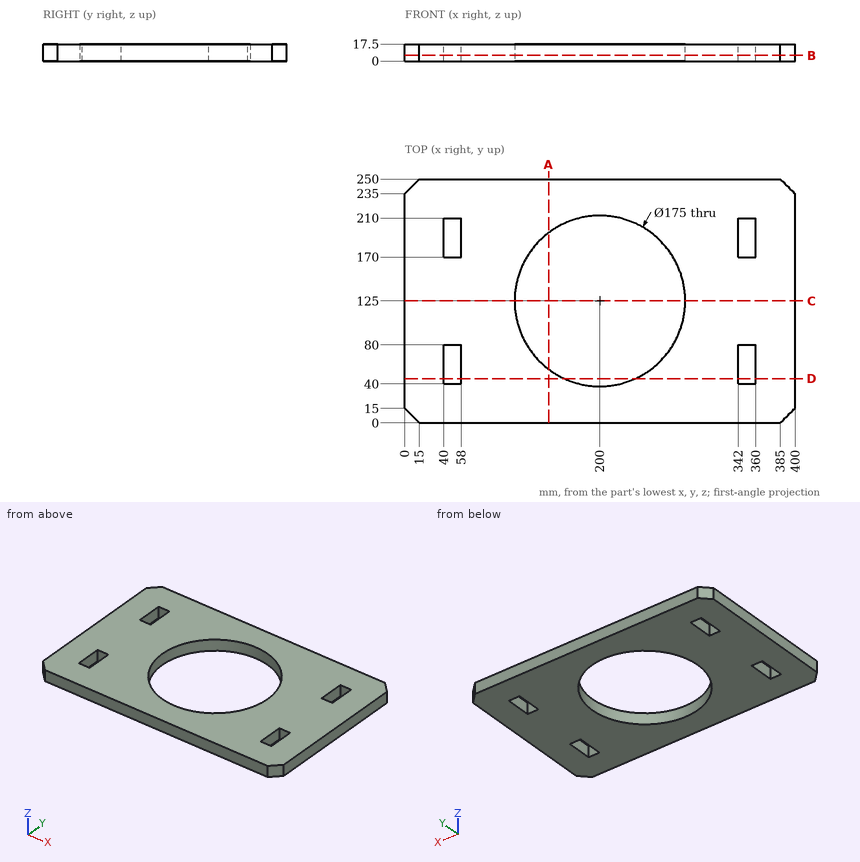
Answer from the drawing. Dimensions are ordinates in mm from the lowest x, y and z of the part. Round coordinates to 2 decimals unless told otherwise and drop trailing zeros. Write each loop counter-clockwise with the first axis right and the second up, starting at its lowest first coordinate (ties: lowest second). Pieces come first, ordered by that corner, then holes. Notation, with made-up numbers: M -18,-4 L 24,-4 A24 cw 24,26 Z; hole C -38.5,30 d6. An arc over 180 degrees is marked long. Write each question's results on one line, items separated by ' | '. Start each with the question number.
Item 1: A cutting plane is placed at B-B on z = 5.75. Write down the section's boundary in (x, y), and give its area (3 significant figures).
Item 2: A cutting plane is placed at C-C on y = 125. Write down the section's boundary in (x, z).
Item 3: A cutting plane is placed at A-A on x = 147.5. Write down the section's boundary in (y, z).
Item 4: A cutting plane is placed at D-D on y = 45.5. Write down the section's boundary in (x, z).
Item 5: Straight lines are drawn through the part: L1, parallel to Y at x = 50.5, z = 7; L2, parallel to X at y = 203, z = 11.5; L3, parallel to Y at x = 200, z = 9.75. For each, find the intervals that lie inside material, in ascending order. Write a range as [from, to].
Check sheet entries:
1) outline: M 0,15 L 15,0 L 385,0 L 400,15 L 400,235 L 385,250 L 15,250 L 0,235 Z; hole M 40,40 L 58,40 L 58,80 L 40,80 Z; hole M 40,170 L 58,170 L 58,210 L 40,210 Z; hole C 200,125 d175; hole M 342,40 L 360,40 L 360,80 L 342,80 Z; hole M 342,170 L 360,170 L 360,210 L 342,210 Z | area: 72,600 mm²
2) outline: M 0,0 L 112.5,0 L 112.5,17.5 L 0,17.5 Z; M 287.5,0 L 400,0 L 400,17.5 L 287.5,17.5 Z
3) outline: M 0,0 L 55,0 L 55,17.5 L 0,17.5 Z; M 195,0 L 250,0 L 250,17.5 L 195,17.5 Z
4) outline: M 0,0 L 40,0 L 40,17.5 L 0,17.5 Z; M 58,0 L 163.45,0 L 163.45,17.5 L 58,17.5 Z; M 236.55,0 L 342,0 L 342,17.5 L 236.55,17.5 Z; M 360,0 L 400,0 L 400,17.5 L 360,17.5 Z
5) L1: [0, 40], [80, 170], [210, 250] | L2: [0, 40], [58, 160.35], [239.65, 342], [360, 400] | L3: [0, 37.5], [212.5, 250]
